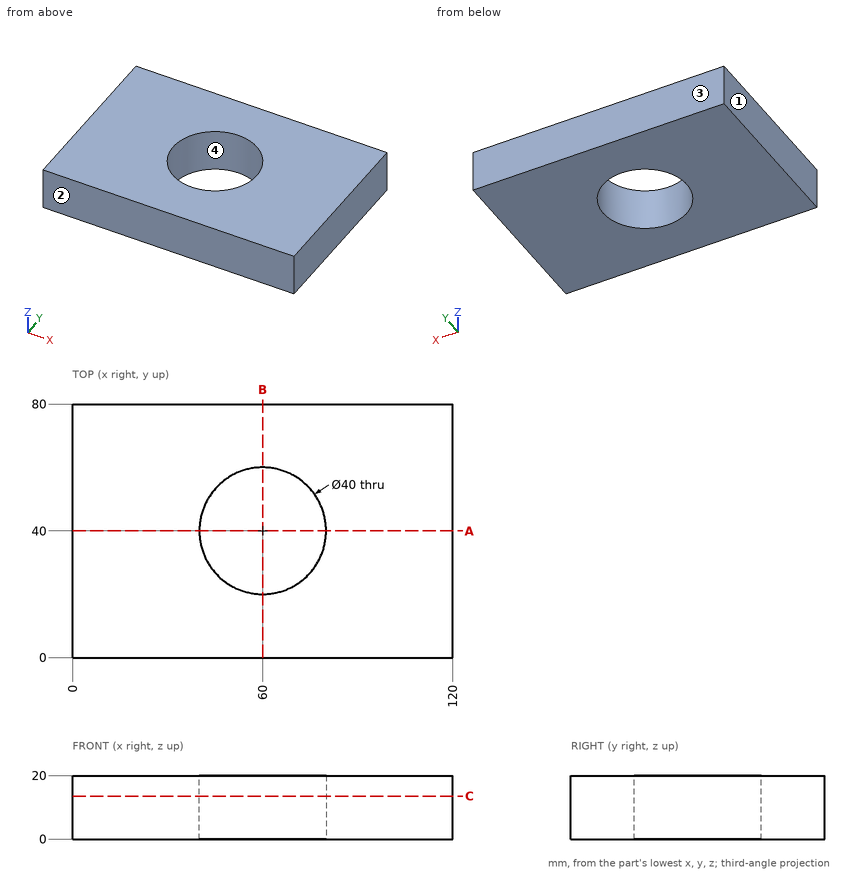
Verification items for this drawing (mm, ordinates from the low corner). Coordinates: 2 decimals unless noted, no trailing zeros. Order: outer loops, then holes, each group sorted by start corner. A loop starts at its lowest first (then second) coordinate and runs counter-clockwise, first axis right, second up. Notation, with made-up numbers: (65, -38.75) - (75, -38.75) arc R5 ccw to (75, -32.75) - close; hole circle Ø4 at (-15, -1). An arc over 180 degrees is marked (long way). Answer as a JSON object with one key per item and string values. Group by question number.
Item 1: Depth check by flat-ended pin: pin 1 Ø12 at (x, y) = (52.5, 23) entering from -Z. Enter the tip coordinate at first touch or a pass-through.
Item 2: Scan lines: probe 1 along Y at (x, z) = (60, 12.25); probe 2 along X at (y, z) = (28.5, 2.75); probe 3 along X at (y, z) = (54, 4). Record each from-to range of solid material in increasing order.
Item 3: Sectioned sample at B-B, the plane x = 60. Record the cut outline in (y, z), and give its area (3 significant figures).
Item 4: Sectioned sample at C-C, the plane z = 13.5. Record the cut outline in (x, y).
Item 5: Draft check along Y on the marked faces 1, 2, 3 and 4. Enter one of: +Y half, -Y half, draft (parallel to the pull), parting line (faces both ways), or undercut.
Item 6: Sectioned sample at A-A, the plane y = 40. Record the cut outline in (x, z), and give its area (3 significant figures).
Resolved:
{
 "1": {"pin 1": "z = 0"},
 "2": {"probe 1": "0 to 20, 60 to 80", "probe 2": "0 to 43.64, 76.36 to 120", "probe 3": "0 to 45.72, 74.28 to 120"},
 "3": {"outline": "(0, 0) - (20, 0) - (20, 20) - (0, 20) - close; (60, 0) - (80, 0) - (80, 20) - (60, 20) - close", "area": "800 mm^2"},
 "4": {"outline": "(0, 0) - (120, 0) - (120, 80) - (0, 80) - close; hole circle Ø40 at (60, 40)"},
 "5": {"face 1": "draft", "face 2": "-Y half", "face 3": "+Y half", "face 4": "undercut"},
 "6": {"outline": "(0, 0) - (40, 0) - (40, 20) - (0, 20) - close; (80, 0) - (120, 0) - (120, 20) - (80, 20) - close", "area": "1,600 mm^2"}
}
